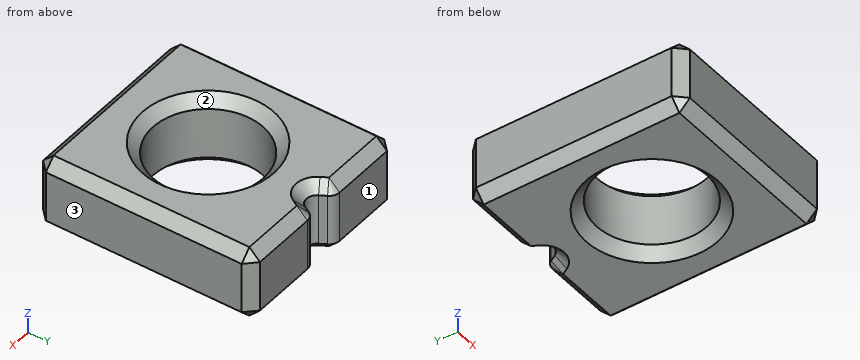
```python
from build123d import *

# Parameters (mm, degrees)
SKETCH101_W     = 9.2
SKETCH101_H     = 3.4
PAD021_DEPTH    = 10.25
SKETCH098_R     = 0.5
POCKET040_DEPTH = 3.401
SKETCH100_R     = 2.6
POCKET041_DEPTH = 3.401
POCKET042_DEPTH = 3.401
FILLET001_R     = 0.5
CHAMFER040_SIZE = 0.5


with BuildPart() as part:
    # Sketch101 → Pad021 (new body)
    with BuildSketch(Plane.XZ):
        Rectangle(SKETCH101_W, SKETCH101_H)
    extrude(amount=PAD021_DEPTH)

    # Sketch098 (on Face1 of Pad021) → Pocket040 (cut, through all)
    with BuildSketch(Plane(origin=(0, 0, -1.7), x_dir=(1, 0, 0), z_dir=(0, 0, -1))):
        with Locations((0, 5.45)):
            Circle(SKETCH098_R)
    extrude(amount=-POCKET040_DEPTH, mode=Mode.SUBTRACT)

    # Sketch100 (on Face7 of Pocket040) → Pocket041 (cut, through all)
    with BuildSketch(Plane(origin=(0, 0, 1.7), x_dir=(-1, 0, 0), z_dir=(0, 0, 1))):
        with Locations((0, 5.45)):
            Circle(SKETCH100_R)
    extrude(amount=-POCKET041_DEPTH, mode=Mode.SUBTRACT)

    # Sketch103 → Pocket042 (cut, through all)
    with BuildSketch(Plane(origin=(0, 0, 1.7), x_dir=(-1, 0, 0), z_dir=(0, 0, 1))):
        Polygon((0.75, 0), (0, 1.299038), (-0.75, 0), align=None)
    extrude(amount=-POCKET042_DEPTH, mode=Mode.SUBTRACT)

    # Fillet001
    fillet001_edges = [part.edges().sort_by_distance(p)[0] for p in [
        (0.75, 0, 0),
        (0, -1.299038, 0),
        (-0.75, 0, 0),
    ]]
    fillet(fillet001_edges, radius=FILLET001_R)

    # Chamfer040
    chamfer040_edges = [part.edges().sort_by_distance(p)[0] for p in [
        (2.819338, 0, 1.7),
        (2.819338, 0, -1.7),
        (4.6, -5.125, -1.7),
        (4.6, -5.125, 1.7),
        (4.6, 0, 0),
        (4.6, -10.25, 0),
        (0, -10.25, -1.7),
        (0, -10.25, 1.7),
        (-4.6, -10.25, 0),
        (-4.6, -5.125, 1.7),
        (-4.6, -5.125, -1.7),
        (-4.6, 0, 0),
        (2.6, -5.45, 1.7),
        (2.6, -5.45, -1.7),
    ]]
    chamfer(chamfer040_edges, length=CHAMFER040_SIZE)


with BuildPart() as part_1:
    # Body020 placement: moved
    add(part.part.moved(Location((15, 20, 2))))


solid = part_1.part
```
Read the model definition and answer for the solid it produces. Units are mm, in the model's axes. Face numbers are marked on the shaded views. Give positions to 0.01 mm unless a question says otherwise; leave off trailing zeros. Write each loop counter-clockwise with the first axis right and the second up, starting at its lowest first coordinate (ties: lowest second). Pieces come first, ordered by that corner, then holes. Notation, with made-up numbers: (-38.75, 21) -> (-22.75, 21) arc R36 ccw to (-22.75, 58) -> close; hole circle Ø7 at (86, 30.5). An arc over 180 degrees is marked (long way). Answer as a JSON object with one key per item and string values.
1) For a pull along Y with two mould halves and no side action, classify the marked faces 1, 2 and 3 as pulls with the +Y half, pulls with the -Y half, needs draft (parallel to the pull), parting line crosses it, or undercut.
Findings below:
{"face 1": "pulls with the +Y half", "face 2": "undercut", "face 3": "needs draft"}
2) Section A-A on x = 15 is taken. Write down the section's boundary in (y, z), then the cut area to 3 significant figures.
Findings below:
{"outline": "(9.75, 0.8) -> (10.25, 0.3) -> (11.45, 0.3) -> (11.95, 0.8) -> (11.95, 3.2) -> (11.45, 3.7) -> (10.25, 3.7) -> (9.75, 3.2) -> close; (17.15, 0.8) -> (17.65, 0.3) -> (18.7, 0.3) -> (19.2, 0.8) -> (19.2, 3.2) -> (18.7, 3.7) -> (17.65, 3.7) -> (17.15, 3.2) -> close", "area": "13.5 mm^2"}
3) Straight lines are drawn through the part: probe 1 along X at (y, z) = (14.55, 1.8); probe 2 along Y at (x, z) = (15, 2.4); probe 3 along X at (y, z) = (16, 1.25). For each, find the intervals that lie inside material, in ascending order. Write a range as from..to.
Findings below:
{"probe 1": "x = 10.4..12.4, 17.6..19.6", "probe 2": "y = 9.75..11.95, 17.15..19.2", "probe 3": "x = 10.4..12.84, 17.16..19.6"}
4) Section B-B on z = 2.3 is taken. Write down the section's boundary in (x, y), then the cut area to 3 significant figures.
Findings below:
{"outline": "(10.4, 10.25) -> (10.9, 9.75) -> (19.1, 9.75) -> (19.6, 10.25) -> (19.6, 19.5) -> (19.1, 20) -> (16.04, 20) arc R0.5 ccw to (15.61, 19.75) -> (15.43, 19.45) arc R0.5 cw to (14.57, 19.45) -> (14.39, 19.75) arc R0.5 ccw to (13.96, 20) -> (10.9, 20) -> (10.4, 19.5) -> close; hole circle Ø5.2 at (15, 14.55)", "area": "71.7 mm^2"}
5) Section C-C on y = 14.55 is taken. Write down the section's boundary in (x, z), then the cut area to 3 significant figures.
Findings below:
{"outline": "(10.4, 0.8) -> (10.9, 0.3) -> (11.9, 0.3) -> (12.4, 0.8) -> (12.4, 3.2) -> (11.9, 3.7) -> (10.9, 3.7) -> (10.4, 3.2) -> close; (17.6, 0.8) -> (18.1, 0.3) -> (19.1, 0.3) -> (19.6, 0.8) -> (19.6, 3.2) -> (19.1, 3.7) -> (18.1, 3.7) -> (17.6, 3.2) -> close", "area": "12.6 mm^2"}
